Read the model definition and answer for the solid it produces. Units are mm, in the model's axes. A direction names the side the tool comes from. Coordinates: 2 decimals unless noted, no trailing zeros. Order: outer loops, then holes, each group sorted by start corner. A loop starts at its lowest first (then second) coordinate and runs counter-clockwise, first axis right, second up. Notation, with made-up numbers: (23.25, 18.25) - (57.25, 18.25) arc R13 cw to (57.25, 26.25) - close; hole circle Ø8 at (-35, 0). An arc over 180 degrees is marked (long way). Use one line per item in the form item = value. Start each with the question number.
from build123d import *

# Parameters (mm, degrees)
F0_W      = 100
F0_H      = 100
F1_DEPTH  = 100
F2_W      = 25
F2_H      = 25
F3_DEPTH  = 25
F4_DEPTH  = 15
F5_DEPTH  = 10
F6_DEPTH  = 5
F8_DEPTH  = 5
F9_W      = 15
F9_H      = 15
F10_DEPTH = 20
F11_W     = 10
F11_H     = 10
F12_DEPTH = 5


with BuildPart() as f1:
    # F0 (on Top) → F1 (new body)
    with BuildSketch(Plane.XY):
        with Locations((1.3461533941, 0)):
            Rectangle(F0_W, F0_H)
    extrude(amount=F1_DEPTH)

    # F2 (on face) → F3 (cut)
    with BuildSketch(Plane(origin=(-48.6538466059, 0, 0), x_dir=(0, -1, 0), z_dir=(-1, 0, 0))):
        with Locations((-37.5, 87.5)):
            Rectangle(F2_W, F2_H)
        with Locations((-37.5, 12.5)):
            Rectangle(F2_W, F2_H)
        with Locations((37.5, 12.5)):
            Rectangle(F2_W, F2_H)
        with Locations((37.5, 87.5)):
            Rectangle(F2_W, F2_H)
    extrude(amount=-F3_DEPTH, mode=Mode.SUBTRACT)

    # F2 (on face) → F4 (cut)
    with BuildSketch(Plane(origin=(-48.6538466059, 0, 0), x_dir=(0, -1, 0), z_dir=(-1, 0, 0))):
        with Locations((-37.5, 62.5)):
            Rectangle(F2_W, F2_H)
        with Locations((37.5, 37.5)):
            Rectangle(F2_W, F2_H)
        with Locations((12.5, 87.5)):
            Rectangle(F2_W, F2_H)
        with Locations((-12.5, 12.5)):
            Rectangle(F2_W, F2_H)
    extrude(amount=-F4_DEPTH, mode=Mode.SUBTRACT)

    # F2 (on face) → F5 (cut)
    with BuildSketch(Plane(origin=(-48.6538466059, 0, 0), x_dir=(0, -1, 0), z_dir=(-1, 0, 0))):
        with Locations((-12.5, 87.5)):
            Rectangle(F2_W, F2_H)
        with Locations((12.5, 12.5)):
            Rectangle(F2_W, F2_H)
        with Locations((-37.5, 37.5)):
            Rectangle(F2_W, F2_H)
        with Locations((37.5, 62.5)):
            Rectangle(F2_W, F2_H)
    extrude(amount=-F5_DEPTH, mode=Mode.SUBTRACT)

    # F2 (on face) → F6 (cut)
    with BuildSketch(Plane(origin=(-48.6538466059, 0, 0), x_dir=(0, -1, 0), z_dir=(-1, 0, 0))):
        with Locations((12.5, 62.5)):
            Rectangle(F2_W, F2_H)
    extrude(amount=-F6_DEPTH, mode=Mode.SUBTRACT)

    # F7 (on face) → F8 (cut)
    with BuildSketch(Plane.XY.offset(100)):
        Polygon((-13.6538466059, 44.5087721944), (-13.6538466059, 50), (-23.6538466059, 50), (-23.6538466059, 34.5087721944), (-10, 34.5087721944), (-10, 20.8771936595), (31.8771933764, 20.8771936595), (31.8771933764, 4.2982455343), (51.3461533941, 4.2982455343), (51.3461533941, 14.2982455343), (41.8771933764, 14.2982455343), (41.8771933764, 30.8771936595), (0, 30.8771936595), (0, 44.5087721944), align=None)
    extrude(amount=-F8_DEPTH, mode=Mode.SUBTRACT)

    # F9 (on face) → F10 (join)
    with BuildSketch(Plane.XY.offset(100)):
        with Locations((16.3082494724, 0)):
            Rectangle(F9_W, F9_H)
    extrude(amount=F10_DEPTH)

    # F11 (on face) → F12 (join)
    with BuildSketch(Plane.XY.offset(120)):
        with Locations((16.3082494724, 0)):
            Rectangle(F11_W, F11_H)
    extrude(amount=F12_DEPTH)


solid = f1.part
Q1. Consider probe 1 along Y at (x, z) = (37.5, 96); probe 2 along X at (y, z) = (-38.5, 83.5); probe 3 along Z at (x, y) = (38, 43). Determine where each line is inside the solid, lowest interval first.
Q2. A cutting plane is placed at B-B (z = 41). Give the vertices of the cut face in (x, y).
Q3. A cutting plane is placed at A-A (x = -32). Give the vertices of the cut face in (y, z), then the cut area to 3 significant figures.
Q4. A cutting plane is placed at D-D (x = -5.5). Give the vertices of the cut face in (y, z).
Q5. Which of the six approach directions +Z, -Z, +X, -X, +Y, -Y give full straight-line access (tool end or side, diameter ignored) to faces 4 (the flat face through (16, -5, 122)), 5 (the flat face through (-36, 0, 12)), 6 (the flat face through (-23.654, 38, 85)), 7 (the flat face through (-7, 44.509, 98)), 8 (the flat face through (-29, -25, 87))?
Q6. Given P1, Ø12.5, axis at y = 32.5, z = 35.5, coming from the -X side; P2, Ø1.5, axis at x = -29.5, z = 21.5, coming from the -Y side; P3, Ø11, axis at x = -31, y = -34.5, coming from the -Z side, each flat-ended and moving along its own axis, determine where each tip first touches the part or whether it passes through.
Q7. A cutting plane is placed at C-C (y = -18.5). Give the vertices of the cut face in (x, z), then the cut area to 3 significant figures.
Q8. For a pull along X with two mould halves and no side action, classify faces 1 (the flat face through (-38.654, -37, 63)), 2 (the flat face through (-10, 28, 98)), 3 (the flat face through (11, 0, 120)) as +X half, -X half, draft (parallel to the pull), parting line (faces both ways), or undercut.
Result sheet:
q1.probe_1 = -50 to 4.3, 30.88 to 50
q1.probe_2 = -23.65 to 51.35
q1.probe_3 = 0 to 100
q2.outline = (-48.65, -25) - (-33.65, -25) - (-33.65, -50) - (51.35, -50) - (51.35, 50) - (-38.65, 50) - (-38.65, 25) - (-48.65, 25) - close
q3.outline = (-50, 25) - (-25, 25) - (-25, 0) - (25, 0) - (25, 25) - (50, 25) - (50, 75) - (25, 75) - (25, 100) - (-25, 100) - (-25, 75) - (-50, 75) - close
q3.area = 7,500 mm^2
q4.outline = (-50, 0) - (50, 0) - (50, 100) - (44.51, 100) - (44.51, 95) - (20.88, 95) - (20.88, 100) - (-50, 100) - close
q5.face_4 = +Z, +X, -X, -Y
q5.face_5 = -Z, -X, +Y
q5.face_6 = +Z, -X, +Y
q5.face_7 = +Z, -X
q5.face_8 = +Z, -X, -Y
q6.P1 = -38.65
q6.P2 = -25
q6.P3 = 25
q7.outline = (-48.65, 25) - (-38.65, 25) - (-38.65, 0) - (51.35, 0) - (51.35, 100) - (-33.65, 100) - (-33.65, 75) - (-43.65, 75) - (-43.65, 50) - (-48.65, 50) - close
q7.area = 9,250 mm^2
q8.face_1 = -X half
q8.face_2 = undercut
q8.face_3 = draft
